Autodesk Inventor part; units mm, degrees
ref_plane "YZ Plane" through (0, 0, 0) normal (1, 0, 0) x (0, 1, 0)
ref_plane "XZ Plane" through (0, 0, 0) normal (0, 1, 0) x (-1, 0, 0)
ref_plane "XY Plane" through (0, 0, 0) normal (0, 0, 1) x (1, 0, 0)
sketch "Sketch1" plane through (0, 0, 0) normal (0, 0, 1) x (1, 0, 0)
  line L0 (0, 0) -> (1, 0)
  line L1 (0.5, 0) -> (0.5, 15.3)
  line L2 (0.5, 0) -> (15.8, 0) construction
  line L3 (0, 15.3) -> (1, 15.3)
  line L4 (1, 0) -> (2.1839, 4.7541)
  line L5 (2.1839, 4.7541) -> (2.5706, 8.6743)
  line L6 (1, 15.3) -> (1.9212, 12.0419)
  line L7 (1.9212, 12.0419) -> (2.5706, 8.6743)
  line L8 (0, 15.3) -> (0.9212, 12.0419)
  line L9 (0.9212, 12.0419) -> (1.5706, 8.6743)
  line L10 (1.1839, 4.7541) -> (1.5706, 8.6743)
  line L11 (0, 0) -> (1.1839, 4.7541)
  point P0 (0.5, 0)
  point P1 (0.5, 15.3)
  dimension "d0" = 1
  dimension "d1" = 15.3
  dimension "d2" = 90
  dimension "d4" = 0
  dimension "d5" = 1
  dimension "d6" = 0.5
extrude "Extrusion1" add sketch "Sketch1" along normal blind 1 contours L11 L1 L0 | L1 L11 L10 L9 L8 L3 L6 L7 L5 L4 L0 | L8 L3 L1
sketch "Sketch2" plane through (-0.71, 15.3, 0) normal (0, 1, 0) x (1, 0, 0)
  line L0 (1.71, 0) -> (0.71, 0)
  line L1 (1.71, -1) -> (0.71, -1)
  line L2 (1.71, 0) -> (1.71, -1)
  line L3 (0.71, 0) -> (0.71, -1)
extrude "Extrusion2" add sketch "Sketch2" along normal blind 4
sketch "Sketch4" plane through (1, 15.3, 0) normal (1, 0, 0) x (0, 0, -1)
  line L0 (-1, 4) -> (0, 4)
  line L1 (-1, -15.3) -> (0, -15.3)
  line L2 (4.3, -20.4) -> (3.7812, -18.7843)
  line L3 (3.7812, -18.7843) -> (2.1719, -17.398)
  line L4 (2.1719, -17.398) -> (0.4286, -17.1646)
  line L5 (0.4286, -17.1646) -> (-0.5, -16.2449)
  line L6 (-0.5, -16.2449) -> (-1, -15.3)
  line L7 (5.3, -20.4) -> (4.5609, -18.2271)
  line L8 (4.5609, -18.2271) -> (2.7638, -16.6488)
  line L9 (2.7638, -16.6488) -> (0.7923, -16.3849)
  line L10 (0.7923, -16.3849) -> (0.3338, -15.9308)
  line L11 (0.3338, -15.9308) -> (0, -15.3)
  line L12 (4.3, -20.4) -> (5.3, -20.4)
  line L13 (0, -15.3) -> (-1, -15.3)
  point P0 (0, 3)
  point P1 (0, -15.3)
  dimension "d13" = 1
  dimension "d22" = 5.1
  dimension "d23" = 5.1
  dimension "d24" = 5.3
  dimension "d25" = 5.3
  dimension "d28" = 0
  dimension "d29" = 0
extrude "Extrusion4" add sketch "Sketch4" against normal blind 1
sketch "Sketch6" plane through (1, -5.1, -5.3) normal (0, -1, 0) x (1, 0, 0)
  line L0 (0, 1) -> (0, 0)
  line L1 (0, 1) -> (-1, 1)
  line L2 (-1, 0) -> (-1, 1)
  line L3 (0, 0) -> (-1, 0)
  point P0 (-1, 5.3)
extrude "Extrusion6" add sketch "Sketch6" along normal blind 1
equation "\"d23\" = d22"
equation "\"d25\" = d24"
properties part number "jst-vh-2p_wire"
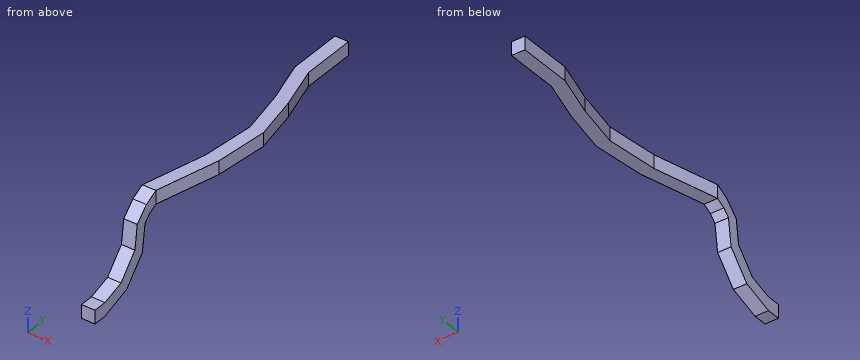
Work out the finished part from the listing and answer in its coordinate system (mm). Round coordinates to 2 decimals unless told otherwise and drop trailing zeros. Write each loop counter-clockwise with the first axis right and the second up, starting at its lowest first coordinate (ties: lowest second). Pieces come first, ordered by that corner, then holes. Notation, with made-up numbers: (57.5, -23) -> (95.5, -23) arc R30 cw to (95.5, 14) -> close; hole circle Ø4 at (78.25, 54). An arc over 180 degrees is marked (long way). Write each question's results on one line, items separated by ' | '.
1) The part is cut by section B-B (z = -3.5). Write down the section's boundary in (x, y).
Findings:
outline: (0, -3.24) -> (1, -3.24) -> (1, -2) -> (0, -2) -> close
2) The part is cut by section C-C (y = 15). Write down the section's boundary in (x, z).
Findings:
outline: (0.08, 0) -> (1.08, 0) -> (1.08, 1) -> (0.08, 1) -> close
3) Consider line 1 along Z through (x, y) = (0.85, 13.5); line 2 along Y through (x, z) = (0.6, -0.25); line 3 along Z through (x, y) = (0.4, -1). Determine where each line is inside the solid, lowest interval first. Write a range as [from, to].
Findings:
line 1: z = [0, 1] | line 2: y = [-1.69, -0.47] | line 3: z = [-0.71, 0.44]
4) The part is cut by section A-A (x = 0.4). Write down the section's boundary in (y, z), and give its area (3 significant figures).
Findings:
outline: (-6.1, -5.3) -> (-5.1, -5.3) -> (-2.93, -4.56) -> (-1.35, -2.76) -> (-1.08, -0.79) -> (-0.63, -0.33) -> (0, 0) -> (1.61, 0) -> (1.61, 1) -> (0, 1) -> (-0.94, 0.5) -> (-1.86, -0.43) -> (-2.1, -2.17) -> (-3.48, -3.78) -> (-5.1, -4.3) -> (-6.1, -4.3) -> close; (13.89, 0) -> (19.3, 0) -> (19.3, 1) -> (13.89, 1) -> close | area: 15.1 mm²
5) Flat-ended cylindrical pins translate along their axes: pin 1 (0.5 mm diameter, centred on y = 17.5, z = 0.5, fed in from +X); pin 2 (0.8 mm diameter, centred on x = 1.5, y = 8, fed in from -Z). Find the tip coordinate at first contact, or state that the pin passes through.
Findings:
pin 1: stops at x = 1 | pin 2: stops at z = 0
